Geometry: see drawing. Coordinates: mm, zero at the bounding-box minimum. Round coordinates to 2 decimals unless told otherwise and drop trailing zeros. Write each loop counter-clockwise with the first axis right and the second up, starting at its lowest first coordinate (ties: lowest second). Pieces come first, ordered by that corner, then holes.
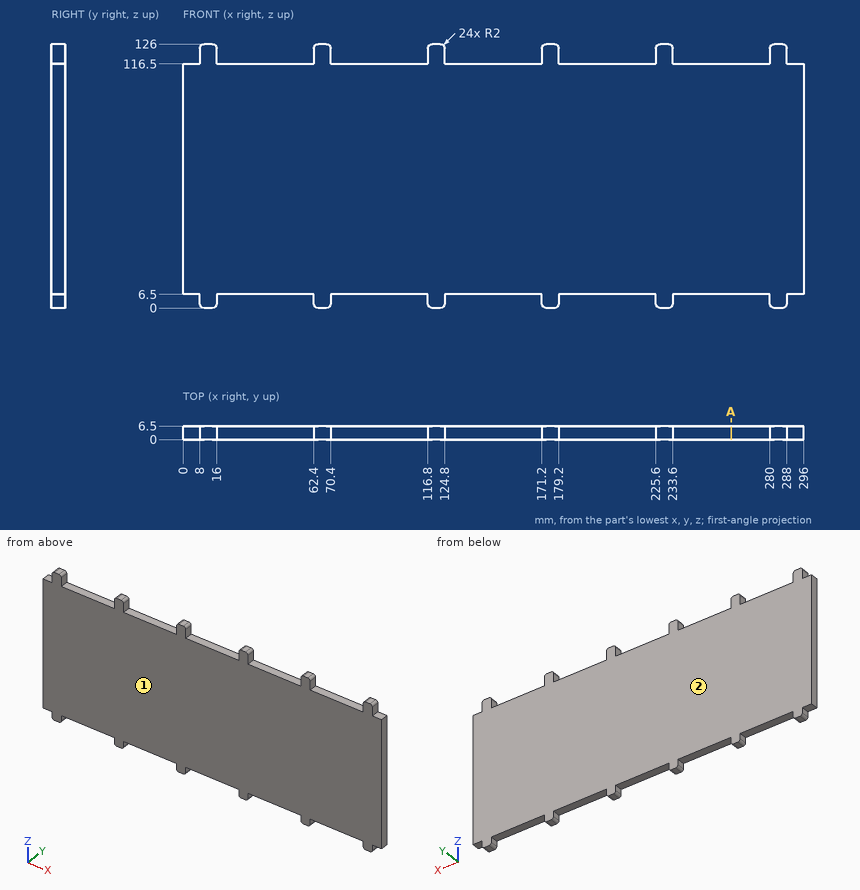
1) Contact query for flat-ended pins moving along their axis: P1, Ø2, axis at y = 3.5, z = 120.5, coming from the +X side; P2, Ø3, axis at x = 210, y = 2.5, coming from the -Z side; P3, Ø1.3, axis at y = 3, z = 3, coming from the -X side. Output: stop coordinate, or through.
Taken from the geometry:
P1: stops at x = 288
P2: stops at z = 6.5
P3: stops at x = 8
2) Pull-direction query (Y, two-part tool) for the marked faces 1 and 2; classes: released by +Y, released by -Y, zero draft, split by the parting line, or undercut.
Taken from the geometry:
face 1: released by -Y
face 2: released by +Y
3) Section query A-A on x = 261.5. Return the cut outline in (y, z), then the cut area to 3 significant figures.
Taken from the geometry:
outline: (0, 6.5) - (6.5, 6.5) - (6.5, 116.5) - (0, 116.5) - close
area: 715 mm2
4) Material intervals for line 1 (Z direction, x = 153, y = 2.5); line 2 (Z direction, x = 63, y = 2), sorted ascending.
Taken from the geometry:
line 1: z = 6.5 to 116.5
line 2: z = 0.57 to 125.43
